Part model, mm, in its own coordinate system. A direction names the side the tool comes from. Give positions to 0.01 mm unless a question says otherwise; leave off trailing zeros. Loops run counter-clockwise (first coordinate to the right, second up) from the corner with the lowest first, then second, coordinate; pieces in that order, holes last. Notation, with made-up numbers: M 26.25,-17 L 85.25,-17 A33 cw 85.25,18 Z; hole C -31.5,28.25 d1. An arc over 180 degrees is marked long. Answer in a Markdown table with one row per item.
from build123d import *

# Parameters (mm, degrees)
BOX018_W                = 12
BOX018_H                = 6
BOX018_DEPTH            = 4.5
CYLINDER020_R           = 2.5
CYLINDER020_DEPTH       = 2
CYLINDER020_PITCH_ANGLE = 90


with BuildPart() as obj1:
    # Box018 → Box018 (new body)
    with BuildSketch(Plane.XY.offset(18)):
        with Locations((6, 3)):
            Rectangle(BOX018_W, BOX018_H)
    extrude(amount=BOX018_DEPTH)


with BuildPart() as audio_jack001:
    # Cylinder020 → Cylinder020 (new body)
    with BuildSketch(Plane.XY):
        Circle(CYLINDER020_R)
    extrude(amount=CYLINDER020_DEPTH)


with BuildPart() as audio_jack001_1:
    # Cylinder020 pitch: moved
    add(audio_jack001.part.rotate(Axis((0, 0, 0), (0, 1, 0)), CYLINDER020_PITCH_ANGLE))


with BuildPart() as audio_jack001_2:
    # Cylinder020 placement: moved
    add(audio_jack001_1.part.moved(Location((12, 3, 20.3))))

    # Fusion011: union obj1
    add(obj1.part)


with BuildPart() as audio_jack001_3:
    # Fusion011 placement: moved
    add(audio_jack001_2.part.moved(Location((8, 1.6, -10.5))))


solid = audio_jack001_3.part
(1) Saw through at D-D (x = 20.5). Write the cut outline in (y, z).
Recorded:
| item | result |
|---|---|
| outline | C 4.6,9.8 d5 |
(2) Saw through at C-C (x = 16.25). Write the cut outline in (y, z), plus the area to 3 significant figures.
Recorded:
| item | result |
|---|---|
| outline | M 1.6,7.5 L 7.6,7.5 L 7.6,12 L 1.6,12 Z |
| area | 27.0 mm^2 |
(3) Pin check, flat tips, straight feed: pin 1 Ø1.5 at (x, y) = (16.5, 5) entering from -Z; pin 2 Ø3 at (x, y) = (13.5, 5) entering from +Z. Stop position of each tip, or through.
Recorded:
| item | result |
|---|---|
| pin 1 | stops at z = 7.5 |
| pin 2 | stops at z = 12 |
(4) Drill centre lines: line 1 along Z through (x, y) = (19.5, 5.55); line 2 along X through (y, z) = (2.45, 7.85); line 3 along Z through (x, y) = (21, 6.8). Where is each one in solid material? Low to high.
Recorded:
| item | result |
|---|---|
| line 1 | z = 7.5 to 12 |
| line 2 | x = 8 to 20 |
| line 3 | z = 8.61 to 10.99 |
(5) Which spindle directions (+Z, -Z, +X, -X, +Y, -Y) get a long thin tool onto all of the face, cutting with end or side? Do faces 1 (the face through (14, 5, 7.5)), 2 (the face through (20, 1.9, 9.7)), 3 (the face through (20.99, 6.29, 11.64)). Say none if no direction does.
Recorded:
| item | result |
|---|---|
| face 1 | -Z, -X, +Y, -Y |
| face 2 | +X, -Y |
| face 3 | +X |
(6) Saw through at B-B (y = 4.1). Write the cut outline in (x, z), plus the area to 3 significant figures.
Recorded:
| item | result |
|---|---|
| outline | M 8,7.5 L 20,7.5 L 20,7.35 L 22,7.35 L 22,12.25 L 20,12.25 L 20,12 L 8,12 Z |
| area | 63.8 mm^2 |
(7) Saw through at A-A (z = 9.8). Write the cut outline in (x, y).
Recorded:
| item | result |
|---|---|
| outline | M 8,1.6 L 20,1.6 L 20,2.1 L 22,2.1 L 22,7.1 L 20,7.1 L 20,7.6 L 8,7.6 Z |
